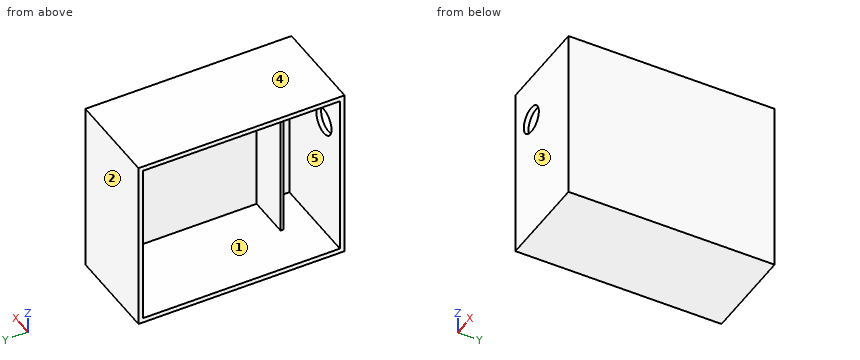
Solid Edge part; units mm, degrees
sketch "Sketch1" plane through (0, 0, 0) normal (1, 0, 0) x (0, 1, 0)
  line L0 (65.5, 55.5) -> (65.5, -55.5)
  line L1 (-65.5, -55.5) -> (65.5, -55.5)
  line L2 (-65.5, 55.5) -> (-65.5, -55.5)
  line L3 (65.5, 55.5) -> (-65.5, 55.5)
extrude "Protrusion1" add sketch "Sketch1" along normal blind 60
shell "Thinwall_3" thickness 3 removed faces 1 at (0, 42.3567, 38.11)
sketch "Sketch2" plane through (60, 0, 0) normal (1, 0, 0) x (0, 0, 1)
  line L0 (-55.5, 43.5) -> (-55.5, 41.6664)
  line L1 (55.5, 43.5) -> (-55.5, 43.5)
  line L2 (55.5, 41.6664) -> (55.5, 43.5)
  line L3 (-55.5, 41.6277) -> (55.5, 41.6664)
extrude "ExtrudedCutout_2" add sketch "Sketch2" against normal blind 30 material side at (60, -42.5832, -55.55)
sketch "Sketch3" plane through (28.5, -62.5, 0) normal (0, 1, 0) x (1, 0, 0)
  circle A0 centre (-10.5, -25.5) radius 8.5
extrude "ExtrudedCutout_4" cut sketch "Sketch3" along normal mid plane 13.736
Source: CAD feature listing. Evaluate the final solid. Frame: model axes, mm. Face numbers are marked on the shaded views. A direction names the side the tool comes from. Give positions to 0.01 mm unless a question says otherwise; leave off trailing zeros. Write each loop counter-clockwise with the first axis right and the second up, starting at its lowest first coordinate (ties: lowest second). Pieces come first, ordered by that corner, then holes. Notation, with made-up numbers: (-15, 64.5) -> (-10, 64.5) arc R16 cw to (-10, 73.5) -> close; hole circle Ø8 at (59.25, 89). An arc over 180 degrees is marked (long way). Return JSON: item names as keys, results as strings. Group by question number.
1. Section A-A, the plane x = 34.5. Output: boundary loops of the cut face in (y, z), then the cut area to 3 significant figures.
2. Material intervals for line 1 (Y direction, x = 36.5, z = -24.5); line 2 (Y direction, x = 28.5, z = -33.5); line 3 (X direction, y = -64.4, z = 25.5), sorted ascending. Write a range as from..to.
3. Mould query, pull axis Y, two halves, no side actions, for the marked faces 3, 4 and 5. Classes: +Y half, -Y half, draft (parallel to the pull), parting line (faces both ways), or undercut.
4. Section C-C, the plane x = 7.5. Output: boundary loops of the cut face in (y, z).
5. Section D-D, the plane x = 18. Output: boundary loops of the cut face in (y, z).
6. Section B-B, the plane z = 25.5. Output: boundary loops of the cut face in (x, y), then the cut area to 3 significant figures.
7. Access query for the marked faces 1 and 2. Directions: +Z, -Z, +X, -X, +Y, -Y. A direction counts if a zero-diameter tool reaches every point of the face in a straight line with its end or side. Return the directions, or none.
8. Pin query (flat end, axial travel): pin 1 Ø8 at (y, z) = (-44, -17) entering from -X; pin 2 Ø1 at (y, z) = (23, -11.5) entering from -X. Return the tip coordinate at first contact, or that it passes through.
Determined:
{
 "1": {"outline": "(-65.5, -55.5) -> (65.5, -55.5) -> (65.5, 55.5) -> (-65.5, 55.5) -> close; hole (-62.5, -52.5) -> (-43.5, -52.5) -> (-43.5, 52.5) -> (-62.5, 52.5) -> close; hole (-41.67, 52.5) -> (-41.63, -52.5) -> (62.5, -52.5) -> (62.5, 52.5) -> close", "area": "1,610 mm2"},
 "2": {"line 1": "y = -65.5..-62.5, -43.5..-41.64, 62.5..65.5", "line 2": "y = -65.5..-62.5, 62.5..65.5", "line 3": "x = 0..9.5, 26.5..60"},
 "3": {"face 3": "-Y half", "face 4": "draft", "face 5": "undercut"},
 "4": {"outline": "(-65.5, -55.5) -> (65.5, -55.5) -> (65.5, 55.5) -> (-65.5, 55.5) -> close; hole (-62.5, -52.5) -> (62.5, -52.5) -> (62.5, 52.5) -> (-62.5, 52.5) -> close"},
 "5": {"outline": "(-65.5, -55.5) -> (65.5, -55.5) -> (65.5, 55.5) -> (-65.5, 55.5) -> (-65.5, 34) -> (-62.5, 34) -> (-62.5, 52.5) -> (62.5, 52.5) -> (62.5, -52.5) -> (-62.5, -52.5) -> (-62.5, 17) -> (-65.5, 17) -> close"},
 "6": {"outline": "(0, -65.5) -> (9.5, -65.5) -> (9.5, -62.5) -> (0, -62.5) -> close; (0, 62.5) -> (57, 62.5) -> (57, -41.66) -> (30, -41.66) -> (30, -43.5) -> (57, -43.5) -> (57, -62.5) -> (26.5, -62.5) -> (26.5, -65.5) -> (60, -65.5) -> (60, 65.5) -> (0, 65.5) -> close", "area": "734 mm2"},
 "7": {"face 1": "-X", "face 2": "+Z, -Z, +X, -X, +Y"},
 "8": {"pin 1": "stops at x = 30", "pin 2": "stops at x = 57"}
}
